Source: CAD feature listing. Evaluate the final solid. Frame: model axes, mm. A direction names the side the tool comes from. Give positions to 0.01 mm unless a question says otherwise; leave off trailing zeros. Write each loop counter-clockwise with the first axis right and the second up, starting at its lowest first coordinate (ties: lowest second). Pieces come first, ordered by that corner, then holes. Notation, with made-up numbers: (22.5, 63) -> (76.5, 63) arc R28 cw to (76.5, 100) -> close; hole circle Ø1 at (-35, 2). An arc over 180 degrees is marked (long way). Use one line per item in the form item = value. Start each with the question number.
(1) Draft query along Y for faces 1 (the face through (-10, 7, -4)), 2 (the face through (1.602, -0.253, 16.117)), 3 (the face through (-11.525, -20.323, 32.972)), 4 (the face through (16.322, -17.394, 33.732)). Return one class per face: pulls with the +Y half, pulls with the -Y half, needs draft (parallel to the pull), parting line crosses it, or undercut.
(2) Cut plane B-B, the plane x = 7. Output: boundary loops of the cut face in (y, z).
(3) Set-up query: faces 5 (the face through (-12.728, 0, 16)), 6 (the face through (-2, -11.463, 13)), 7 (the face through (12.272, 3, 13)), 8 (the face through (11, -13, 31)). Return all of +Z, -Z, +X, -X, +Y, -Y with unobstructed straight access to the full face (end or side cutting, diameter ignored); none if empty.
(4) Cut plane D-D, the plane z = 30. Output: boundary loops of the cut face in (x, y), and give its area (3 significant figures).
(5) First-contact query: P1, Ø7, axis at x = 1.27, y = -0.46, coming from the -Z side; P2, Ø2, axis at x = 1, z = -2.5, coming from the -Y side; P3, Ø10, axis at x = 0, z = 13, coming from the -Y side; P4, Ø1, axis at x = 14, z = 23, coming from the +Y side. Flat tips, straight axial feed; report the tip coordinate or a pass-through.
(6) Cut plane A-A, the plane y = -4. Output: boundary loops of the cut face in (x, z), and give its area (3 significant figures).
(7) Cut plane C-C, the plane z = 13. Output: boundary loops of the cut face in (x, y), and give its area (3 significant figures).
(8) Material intervals for line 1 along Y through (x, z) = (1.5, 7.5); line 2 along X through (y, z) = (5, 18.5); line 3 along Z through (x, y) = (20.5, -8), sorted ascending. Write a range as from..to.
Autodesk Inventor part; units mm, degrees
ref_plane "YZ Plane" through (0, 0, 0) normal (1, 0, 0) x (0, 1, 0)
ref_plane "XZ Plane" through (0, 0, 0) normal (0, 1, 0) x (-1, 0, 0)
ref_plane "XY Plane" through (0, 0, 0) normal (0, 0, 1) x (1, 0, 0)
sketch "Sketch1" plane through (0, 0, 0) normal (0, 0, 1) x (1, 0, 0)
  line L0 (-12.7278, 13.5367) -> (12.2722, 13.5367)
  line L1 (12.2722, 13.5367) -> (12.2722, -11.4633)
  line L2 (12.2722, -11.4633) -> (-12.7278, -11.4633)
  line L3 (-12.7278, -11.4633) -> (-12.7278, 13.5367)
  line L4 (-9.7278, -11.4633) -> (-9.7278, 10.5367)
  line L5 (-9.7278, 10.5367) -> (12.2722, 10.5367)
  point P0 (0, 0)
  point P1 (1.2722, -0.4633)
  dimension "d0" = 25
  dimension "d1" = 25
  dimension "d2" = 3
  dimension "d3" = 3
  dimension "d4" = 11
  dimension "d5" = 11
extrude "Extrusion1" add sketch "Sketch1" along normal blind 35
extrude "Extrusion2" add sketch "Sketch1" against normal blind 4 contours L0 L1 L5 L4 L2 L3
hole "Hole1" at (1.2722, -0.4633, 0) direction (0, 0, 1) diameter 4.5 depth 15 tip angle 118
sketch "Sketch2" plane through (0, 0, 35) normal (0, 0, 1) x (1, 0, 0)
  line L0 (-12.7278, 13.5367) -> (-12.7278, -11.4633)
  line L1 (-12.7278, -11.4633) -> (12.2722, -11.4633)
  line L2 (12.2722, -11.4633) -> (12.2722, 13.5367)
  line L3 (12.2722, 13.5367) -> (-12.7278, 13.5367)
  line L4 (12.2722, 13.5367) -> (12.2722, 10.5367)
  line L5 (12.2722, 13.5367) -> (22.2722, 13.5367)
  line L6 (22.2722, 13.5367) -> (22.2722, -21.4633)
  line L7 (22.2722, -21.4633) -> (-12.7278, -21.4633)
  line L8 (-12.7278, -21.4633) -> (-12.7278, -11.4633)
  point P0 (0, 0)
  point P1 (17.2722, 8.5367)
  point P2 (-7.7278, -16.4633)
  point P3 (16.7722, -15.9633)
  dimension "d17" = 10
  dimension "d18" = 10
  dimension "d21" = 5
  dimension "d22" = 5
  dimension "d23" = 5.5
  dimension "d24" = 5.5
  dimension "d25" = 5
  dimension "d26" = 5
extrude "Extrusion3" add sketch "Sketch2" against normal blind 4 contours L1 L2 L5 L6 L7 L8
hole "Hole2" at (17.2722, 8.5367, 35) at (-7.7278, -16.4633, 35) at (16.7722, -15.9633, 35) direction (0, 0, -1) diameter 3 end through all
chamfer "Chamfer1" distance 1.5 angle 45 3 edges at (-7.7278, -14.9633, 31) (16.7722, -14.4633, 31) (17.2722, 10.0367, 31)
fillet "Fillet1" radius 4 4 edges at (22.2722, -21.4633, 33) (-12.7278, -21.4633, 33) (22.2722, 13.5367, 33) (12.2722, -11.4633, 15.5)
fillet "Fillet2" radius 2 3 edges at (-12.7278, 13.5367, 15.5) (12.2722, 3.0367, 31) (-2.2278, -11.4633, 31)
equation "\"d3\" = d2"
properties part number "3DP_PLA_Sorting_line_base_plate_standoff" material "ABS Plastic"
Geometry says:
q1.face_1 = needs draft
q1.face_2 = undercut
q1.face_3 = pulls with the -Y half
q1.face_4 = undercut
q2.outline = (-21.46, 31) -> (-13.46, 31) arc R2 cw to (-11.46, 29) -> (-11.46, 0) -> (10.54, 0) -> (10.54, -4) -> (13.54, -4) -> (13.54, 35) -> (-21.46, 35) -> close
q3.face_5 = +Z, -Z, -X, +Y, -Y
q3.face_6 = -Z, +X, -X, -Y
q3.face_7 = -Z, +X, +Y, -Y
q3.face_8 = -Z, +X, -Y
q4.outline = (-12.73, -11.73) -> (8.27, -11.73) arc R4.27 ccw to (12.54, -7.46) -> (12.54, 13.54) -> (-10.73, 13.54) arc R2 ccw to (-12.73, 11.54) -> close
q4.area = 634 mm^2
q5.P1 = 0
q5.P2 = 10.54
q5.P3 = -11.46
q5.P4 = through
q6.outline = (-12.73, -4) -> (-9.73, -4) -> (-9.73, 0) -> (12.27, 0) -> (12.27, 29) arc R2 cw to (14.27, 31) -> (22.27, 31) -> (22.27, 35) -> (-12.73, 35) -> close
q6.area = 928 mm^2
q7.outline = (-12.73, -11.46) -> (8.27, -11.46) arc R4 ccw to (12.27, -7.46) -> (12.27, 13.54) -> (-10.73, 13.54) arc R2 ccw to (-12.73, 11.54) -> close; hole circle Ø4.5 at (1.27, -0.46)
q7.area = 605 mm^2
q8.line_1 = -11.46..-2.7, 1.78..13.54
q8.line_2 = -12.73..12.27
q8.line_3 = 31..35
